```python
from build123d import *

# Parameters (mm, degrees)
EXTRUDE_THIN1_START = -5
EXTRUDE_THIN1_DEPTH = 40


with BuildPart() as part:
    # Sketch1 → Extrude-Thin1 (new body)
    with BuildSketch(Plane.XY.offset(EXTRUDE_THIN1_START)):
        with BuildLine():
            Line((0, 54), (521.447237603, 54))
            ThreePointArc((521.447237603, 54), (561.197237603, 93.75), (521.447237603, 133.5))
            Line((521.447237603, 133.5), (314.631190532, 133.5))
            Line((314.631190532, 133.5), (314.631190532, 131.5))
            Line((314.631190532, 131.5), (521.447237603, 131.5))
            ThreePointArc((521.447237603, 131.5), (559.197237603, 93.75), (521.447237603, 56))
            Line((521.447237603, 56), (0, 56))
            Line((0, 56), (0, 54))
        make_face()
    extrude(amount=-EXTRUDE_THIN1_DEPTH)


solid = part.part
```
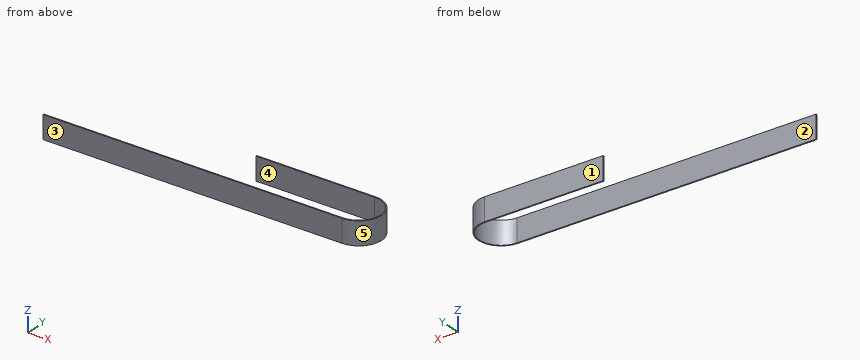
Source: CAD feature listing. Evaluate the final solid. Frame: model axes, mm. Face numbers are marked on the shaded views. A direction names the side the tool comes from. Give positions to 0.01 mm unless a question says otherwise; leave off trailing zeros. Order: outer loops, then holes, each group sorted by start corner. A loop starts at its lowest first (then second) coordinate and runs counter-clockwise, first axis right, second up.
(1) Access query for the marked faces 1 and 2. Directions: +Z, -Z, +X, -X, +Y, -Y. A direction counts if a zero-diameter tool reaches every point of the face in a straight line with its end or side. Return the directions, or none.
(2) Contact query for flat-ended pins moving along their axis: P1, Ø0.6, axis at y = 133, z = -33.5, coming from the -X side; P2, Ø1.5, axis at y = 125, z = -34, coming from the +X side; P3, Ø1.5, axis at y = 104, z = -36, coming from the -X side. Output: stop coordinate, or through.
(3) Pull-direction query (Y, two-part tool) for the marked faces 3, 4 and 5; classes: +Y half, -Y half, draft (parallel to the pull), parting line (faces both ways), or undercut.
(4) Section query C-C (x = 276.5). Return the cut outline in (y, z).
(5) Section query D-D (y = 93.75). Return the cut outline in (x, z), plus the area to 3 significant figures.
(6) Section query B-B (z = -30). Return the cut outline in (x, y).
(7) Section query A-A (x = 385). Return the cut outline in (y, z).
(8) Material intervals for line 1 along Y through (x, z) = (417.5, -18); line 2 along Y through (x, z) = (243, -16.5); line 3 along X through (y, z) = (102, -41), sorted ascending.
Outcome:
1. face 1: +Z, -Z, +X, -X, +Y
1. face 2: +Z, -Z, -X
2. P1: stops at x = 314.63
2. P2: stops at x = 546.94
2. P3: stops at x = 557.56
3. face 3: -Y half
3. face 4: undercut
3. face 5: parting line
4. outline: (54, -45) - (56, -45) - (56, -5) - (54, -5) - close
5. outline: (559.2, -45) - (561.2, -45) - (561.2, -5) - (559.2, -5) - close
5. area: 80.0 mm2
6. outline: (0, 54) - (521.45, 54) arc R39.75 ccw to (521.45, 133.5) - (314.63, 133.5) - (314.63, 131.5) - (521.45, 131.5) arc R37.75 cw to (521.45, 56) - (0, 56) - close
7. outline: (54, -45) - (56, -45) - (56, -5) - (54, -5) - close; (131.5, -45) - (133.5, -45) - (133.5, -5) - (131.5, -5) - close
8. line 1: y = 54 to 56, 131.5 to 133.5
8. line 2: y = 54 to 56
8. line 3: x = 558.28 to 560.33
